```python
from build123d import *

# Parameters (mm, degrees)
F1_DEPTH = 63.5
F2_W     = 38.1
F2_H     = 50.8
F3_DEPTH = 61.976


with BuildPart() as f1:
    # F0 (on Front) → F1 (new body)
    with BuildSketch(Plane.XZ):
        Polygon((-26.163351, 0), (-28.433141, -50.8), (47.766859, -50.8), (47.766859, -25.4), (-3.033141, -25.4), (-3.033141, 25.4), (-66.533141, 25.4), (-66.533141, 0), (-64.263351, 0), align=None)
    extrude(amount=F1_DEPTH)

    # F2 (on face) → F3 (join)
    with BuildSketch(Plane.XZ.offset(63.5)):
        with Locations((16.016859, 0)):
            Rectangle(F2_W, F2_H)
    extrude(amount=-F3_DEPTH)


solid = f1.part
```
Geometry check sheet. Reference: the model listing, model coordinates, mm. A direction names the side the tool comes from. Coordinates: 2 decimals unless noted, no trailing zeros. Order: outer loops, then holes, each group sorted by start corner. A loop starts at its lowest first (then second) coordinate and runs counter-clockwise, first axis right, second up. Notation, with made-up numbers: (76.25, 47) - (105.25, 47) arc R27 cw to (105.25, 83) - close; hole circle Ø9 at (29, 8). An arc over 180 degrees is marked (long way). Answer in a Markdown table with one row per item. Add a question column.
1. Section check C-C (z = 13). Enter the section's corners in (x, y).
2. Material ranges on L1, parallel to Z at x = -58.5, y = -48.5; L2, parallel to Y at x = 7.5, z = 19; L3, parallel to X at y = -21, z = 7.5, recorded low to high. Write a range as [from, to].
3. Section check B-B (x = 0). Enter the section's corners in (y, z).
4. Access from +Z, -Z, +X, -X, +Y, -Y to the whole of each face (thin tool, end or side, straight path). Record for faces 5 (the face through (16, -1.524, 0)), 6 (the face through (3, -63.5, -12)).
5. Gauge pin test, flat ends, axial feed: pin 1 Ø19 at (x, z) = (8.5, 11.5) entering from +Y; pin 2 Ø4 at (y, z) = (-56.5, -7) entering from -X; pin 3 Ø1.2 at (y, z) = (-0.5, 0.5) entering from +X. Record the tip position at first contact, or that the pin passes through.
6. Section check A-A (y = -31.5). Enter the section's corners in (x, z).
7. Section check D-D (x = -51). Enter the section's corners in (y, z), plus the area to 3 significant figures.
8. Draft check along Z on faces 1 (the face through (35.067, -33, 0)), 2 (the face through (-16, -32, 25.4)), 3 (the face through (9, -31, -50.8)), 4 (the face through (-27.282, -31.306, -25.044)). Enter one of: +Z half, -Z half, draft (parallel to the pull), parting line (faces both ways), or undercut.
Data:
| question | item | result |
|---|---|---|
| 1 | outline | (-66.53, -63.5) - (35.07, -63.5) - (35.07, -1.52) - (-3.03, -1.52) - (-3.03, 0) - (-66.53, 0) - close |
| 2 | L1 | z = [0, 25.4] |
| 2 | L2 | y = [-63.5, -1.52] |
| 2 | L3 | x = [-66.53, 35.07] |
| 3 | outline | (-63.5, -50.8) - (0, -50.8) - (0, -25.4) - (-1.52, -25.4) - (-1.52, 25.4) - (-63.5, 25.4) - close |
| 4 | face 5 | +Z, +X, +Y |
| 4 | face 6 | +Z, -Z, +X, -X, -Y |
| 5 | pin 1 | stops at y = -1.52 |
| 5 | pin 2 | stops at x = -26.57 |
| 5 | pin 3 | stops at x = -3.03 |
| 6 | outline | (-66.53, 0) - (-26.16, 0) - (-28.43, -50.8) - (47.77, -50.8) - (47.77, -25.4) - (35.07, -25.4) - (35.07, 25.4) - (-66.53, 25.4) - close |
| 7 | outline | (-63.5, 0) - (0, 0) - (0, 25.4) - (-63.5, 25.4) - close |
| 7 | area | 1,610 mm² |
| 8 | face 1 | draft |
| 8 | face 2 | +Z half |
| 8 | face 3 | -Z half |
| 8 | face 4 | undercut |
